Geometry: final body of the model. Coordinates: model frame, mm. A direction names the side the tool comes from. Coordinates: 2 decimals unless noted, no trailing zeros. Write each loop counter-clockwise with the first axis right and the second up, starting at its lowest first coordinate (ties: lowest second). Pieces come first, ordered by that corner, then holes. Notation, with made-up numbers: (38.5, 48) -> (77.5, 48) arc R23 ccw to (77.5, 59) -> close; hole circle Ø2 at (22, 67.5). An arc over 180 degrees is marked (long way). Answer as a JSON object with one key per item and string values. Group by question number.
```python
from build123d import *

# Parameters (mm, degrees)
SZKIC1_W                    = 100
SZKIC1_H                    = 60
DODANIE_WYCI_GNI_CIE1_DEPTH = 10
SZKIC2_W                    = 100
SZKIC2_H                    = 10
DODANIE_WYCI_GNI_CIE2_DEPTH = 30
OTW_R_POD_RUB_M101_D        = 12
SZYK_LINIOWY2_COUNT         = 2
SZYK_LINIOWY2_PITCH         = 50


with BuildPart() as part:
    # Szkic1 → Dodanie-wyciągnięcie1 (new body)
    with BuildSketch(Plane.XY):
        Rectangle(SZKIC1_W, SZKIC1_H)
    extrude(amount=DODANIE_WYCI_GNI_CIE1_DEPTH)

    # Szkic2 → Dodanie-wyciągnięcie2 (add)
    with BuildSketch(Plane.XY.offset(10)):
        with Locations((0, -25)):
            Rectangle(SZKIC2_W, SZKIC2_H)
    extrude(amount=DODANIE_WYCI_GNI_CIE2_DEPTH)

    # Otwór pod śrubę M101 (through all)
    with Locations(Plane(origin=(0, -20, 0), x_dir=(1, 0, 0), z_dir=(0, 1, 0))):
        with Locations((-25, -25)):
            otw_r_pod_rub_m101 = Hole(OTW_R_POD_RUB_M101_D / 2)

    # Szyk liniowy2: Otwór pod śrubę M101 ×2
    with Locations(*[(i * SZYK_LINIOWY2_PITCH, 0, 0) for i in range(1, SZYK_LINIOWY2_COUNT)]):
        add(otw_r_pod_rub_m101, mode=Mode.SUBTRACT)


solid = part.part
```
Item 1: Ray query, L1, parallel to X at y = -24.75, z = 25; L2, parallel to Z at x = 25, y = -27; L3, parallel to Y at x = -7.5, z = 12. Return the intervals inside material, ascending. Write a range as [from, to].
Item 2: Mould query, pull axis X, two halves, no side actions, for faces 3 (the cylindrical face through (-20.24, -25.07, 28.65)), 4 (the flat face through (-50, -14, 6)), 5 (the flat face through (50, -14, 6)), 6 (the flat face through (-1, 5, 10)). Classes: +X half, -X half, draft (parallel to the pull), parting line (faces both ways), or undercut.
Item 3: Section D-D on y = 9.5. Output: boundary loops of the cut face in (x, z).
Item 4: Section B-B on z = 25. Output: boundary loops of the cut face in (x, y), then the cut area to 3 significant figures.
Item 5: Section C-C on x = 35. Output: boundary loops of the cut face in (y, z).
Item 6: Section A-A on x = 25. Output: boundary loops of the cut face in (y, z).
Item 7: Contact query for flat-ended pins moving along their axis: pin 1 (10 mm diameter, centred on x = -18, y = 8, fed in from +Z); pin 2 (3 mm diameter, centred on x = -5.5, z = 30.5, fed in from +Y); pin 3 (4 mm diameter, centred on y = -19, z = 32.5, fed in from -X); pin 4 (9.5 mm diameter, centred on x = -25, z = 25, fed in from -Y). Output: stop coordinate, or through.
Item 8: Set-up query: faces 1 (the flat face through (-1, -30, 20)), 2 (the flat face through (-1, -20, 25)). Return all of +Z, -Z, +X, -X, +Y, -Y with unobstructed straight access to the full face (end or side cutting, diameter ignored); none if empty.
Answer sheet:
{
 "1": {"L1": "x = [-50, -31], [-19, 19], [31, 50]", "L2": "z = [0, 19], [31, 40]", "L3": "y = [-30, -20]"},
 "2": {"face 3": "undercut", "face 4": "-X half", "face 5": "+X half", "face 6": "draft"},
 "3": {"outline": "(-50, 0) -> (50, 0) -> (50, 10) -> (-50, 10) -> close"},
 "4": {"outline": "(-50, -30) -> (-31, -30) -> (-31, -20) -> (-50, -20) -> close; (-19, -30) -> (19, -30) -> (19, -20) -> (-19, -20) -> close; (31, -30) -> (50, -30) -> (50, -20) -> (31, -20) -> close", "area": "760 mm^2"},
 "5": {"outline": "(-30, 0) -> (30, 0) -> (30, 10) -> (-20, 10) -> (-20, 40) -> (-30, 40) -> close"},
 "6": {"outline": "(-30, 0) -> (30, 0) -> (30, 10) -> (-20, 10) -> (-20, 19) -> (-30, 19) -> close; (-30, 31) -> (-20, 31) -> (-20, 40) -> (-30, 40) -> close"},
 "7": {"pin 1": "stops at z = 10", "pin 2": "stops at y = -20", "pin 3": "stops at x = -50", "pin 4": "passes through"},
 "8": {"face 1": "+Z, -Z, +X, -X, -Y", "face 2": "+Z, +X, -X, +Y"}
}
